```python
from build123d import *

# Parameters (mm, degrees)
F1_DEPTH = 25.4
F3_DEPTH = 25.4


# Not quite as in the source:
# - the program builds the solid bodies; features that only make, move or delete a surface that nothing else refers to are left out


with BuildPart() as f1:
    # F0 (on Front) → F1 (new body)
    with BuildSketch(Plane.XZ):
        with BuildLine():
            ThreePointArc((-73.432606987, 725.1798510551), (0, 728.8883070439), (73.432606987, 725.1798510551))
            Line((73.432606987, 725.1798510551), (885.1755261421, 725.1798510551))
            Line((885.1755261421, 725.1798510551), (885.1755261421, 861.151099205))
            Line((885.1755261421, 861.151099205), (-774.2805480957, 861.151099205))
            Line((-774.2805480957, 861.151099205), (-774.2805480957, 725.1798510551))
            Line((-774.2805480957, 725.1798510551), (-73.432606987, 725.1798510551))
        make_face()
    extrude(amount=F1_DEPTH)

    # F0 (on Front) → F3 (join)
    with BuildSketch(Plane.XZ):
        with BuildLine():
            ThreePointArc((107.6199000481, -720.8995223045), (552.1417620936, -475.8336250177), (728.8883070439, 0))
            ThreePointArc((728.8883070439, 0), (540.7413118737, 488.7504452974), (73.432606987, 725.1798510551))
            Line((73.432606987, 725.1798510551), (-73.432606987, 725.1798510551))
            ThreePointArc((-73.432606987, 725.1798510551), (-728.6846993659, 17.2271023467), (-107.6199000481, -720.8995223045))
            Line((-107.6199000481, -720.8995223045), (107.6199000481, -720.8995223045))
        make_face()
        with BuildLine():
            Line((-73.432606987, 725.1798510551), (73.432606987, 725.1798510551))
            ThreePointArc((73.432606987, 725.1798510551), (0, 728.8883070439), (-73.432606987, 725.1798510551))
        make_face()
        with BuildLine():
            ThreePointArc((-73.432606987, 725.1798510551), (0, 728.8883070439), (73.432606987, 725.1798510551))
            Line((73.432606987, 725.1798510551), (885.1755261421, 725.1798510551))
            Line((885.1755261421, 725.1798510551), (885.1755261421, 861.151099205))
            Line((885.1755261421, 861.151099205), (-774.2805480957, 861.151099205))
            Line((-774.2805480957, 861.151099205), (-774.2805480957, 725.1798510551))
            Line((-774.2805480957, 725.1798510551), (-73.432606987, 725.1798510551))
        make_face()
        with BuildLine():
            Line((885.1755261421, -720.8995223045), (107.6199000481, -720.8995223045))
            ThreePointArc((107.6199000481, -720.8995223045), (0, -728.8883070439), (-107.6199000481, -720.8995223045))
            Line((-107.6199000481, -720.8995223045), (-774.2805480957, -720.8995223045))
            Line((-774.2805480957, -720.8995223045), (-774.2805480957, -838.6484384537))
            Line((-774.2805480957, -838.6484384537), (885.1755261421, -838.6484384537))
            Line((885.1755261421, -838.6484384537), (885.1755261421, -720.8995223045))
        make_face()
        with BuildLine():
            ThreePointArc((-107.6199000481, -720.8995223045), (0, -728.8883070439), (107.6199000481, -720.8995223045))
            Line((107.6199000481, -720.8995223045), (-107.6199000481, -720.8995223045))
        make_face()
    extrude(amount=F3_DEPTH)


solid = f1.part
```
Could you check a few things on this model? Use its own coordinates, in mm. Coordinates: 2 decimals unless noted, no trailing zeros. Loops run counter-clockwise (first coordinate to the right, second up) from the corner with the lowest first, then second, coordinate; pieces in that order, holes last. Notation, with made-up numbers: M -3,-37.5 L 38,-37.5 A27 ccw 38,-11.5 Z; hole C 67.5,85 d2. An arc over 180 degrees is marked long. Put each result on its own line as item: value. Start each with the question number.
(1) Suppose I cut it at B-B on y = -8. Please give me the cut outline in (x, z), then the cut area to 3 significant figures.
(2) Will this pin go through, and if not, where does the flat tip stop? P1, Ø3, axis at y = -23, z = -536, coming from the -X side.
(3) Suppose I cut it at C-C on z = -461.5. Please give me the cut outline in (x, y).
(4) Thinking about a two-plate mould opening in Z: for faces 1 (the face through (-728.187, -12.522, 31.977)), 2 (the face through (44, -25.4, 23)), 3 (the face through (728.884, -12.522, 2.471)), which applies, pulls with the +Z half, pulls with the -Z half, needs draft (parallel to the pull), parting line crosses it, or undercut?
(5) Suppose I cut it at D-D on x = -446. Please give me the cut outline in (y, z), then the cut area to 3 significant figures.
(6) Suppose I cut it at A-A on x = -187. Please give me the cut outline in (y, z).
(7) I need wall thicknesses on line 1 (Z direction, x = 510.5, y = -2); line 2 (Z direction, x = 580.5, y = -23.5); line 3 (Z direction, x = 811, y = -1.5). Which ranges of each line are inside material? Lowest first, please. Write a range as from..to.
Solutions:
1. outline: M -774.28,-838.65 L 885.18,-838.65 L 885.18,-720.9 L 107.62,-720.9 A728.89 ccw 73.43,725.18 L 885.18,725.18 L 885.18,861.15 L -774.28,861.15 L -774.28,725.18 L -73.43,725.18 A728.89 ccw -107.62,-720.9 L -774.28,-720.9 Z
1. area: 2,090,000 mm2
2. P1: stops at x = -495.57
3. outline: M -564.18,-25.4 L 564.18,-25.4 L 564.18,0 L -564.18,0 Z
4. face 1: undercut
4. face 2: needs draft
4. face 3: undercut
5. outline: M -25.4,-838.65 L 0,-838.65 L 0,-720.9 L -25.4,-720.9 Z; M -25.4,-576.51 L 0,-576.51 L 0,576.51 L -25.4,576.51 Z; M -25.4,725.18 L 0,725.18 L 0,861.15 L -25.4,861.15 Z
5. area: 35,700 mm2
6. outline: M -25.4,-838.65 L 0,-838.65 L 0,-720.9 L -25.4,-720.9 Z; M -25.4,-704.49 L 0,-704.49 L 0,704.49 L -25.4,704.49 Z; M -25.4,725.18 L 0,725.18 L 0,861.15 L -25.4,861.15 Z
7. line 1: z = -838.65..-720.9, -520.26..520.26, 725.18..861.15
7. line 2: z = -838.65..-720.9, -440.79..440.79, 725.18..861.15
7. line 3: z = -838.65..-720.9, 725.18..861.15
